from build123d import *

# Parameters (mm, degrees)
F0_R     = 12.7
F1_DEPTH = 1.27
F3_DEPTH = 25.4
F5_W     = 1.905
F5_H     = 31.75
F6_DEPTH = 6.35
F7_R     = 5.08


with BuildPart() as f1:
    # F0 (on Top) → F1 (new body)
    with BuildSketch(Plane.XY):
        Circle(F0_R)
    extrude(amount=F1_DEPTH)

    # F2 (on Top) → F3 (join)
    with BuildSketch(Plane.XY):
        Polygon((19.35988, 12.7), (-19.05, 12.7), (-19.05, -50.8), (-8.7376, -50.8), (-8.7376, -19.05), (9.0424, -19.05), (9.0424, -50.8), (19.35988, -50.8), align=None)
    extrude(amount=-F3_DEPTH)

    # F5 (on face) → F6 (cut)
    with BuildSketch(Plane(origin=(0, 0, -25.4), x_dir=(1, 0, 0), z_dir=(0, 0, -1))):
        with Locations((-9.6901, 34.925)):
            Rectangle(F5_W, F5_H)
        with Locations((9.9949, 34.925)):
            Rectangle(F5_W, F5_H)
    extrude(amount=-F6_DEPTH, mode=Mode.SUBTRACT)

    # F7
    f7_edges = [f1.edges().sort_by_distance(p)[0] for p in [
        (-13.8938, -50.8, 0),
        (-19.05, -50.8, -12.7),
        (14.20114, -50.8, 0),
        (19.35988, -50.8, -12.7),
        (19.35988, 12.7, -12.7),
        (-19.05, 12.7, -12.7),
    ]]
    fillet(f7_edges, radius=F7_R)


solid = f1.part
Part model, mm, in its own coordinate system. A direction names the side the tool comes from. Give positions to 0.01 mm unless a question says otherwise; leave off trailing zeros. Write each loop counter-clockwise with the first axis right and the second up, starting at its lowest first coordinate (ties: lowest second). Pieces come first, ordered by that corner, then holes.
1) Two-plate mould, pull along X, no slides. Class faces 1 (the face through (-2.75, -12.4, 0.63)), 2 (the face through (12, -50.8, -15)), 3 (the face through (17.832, 11.251, -12.878)), 4 (the face through (10, -35, -19.05)): released by +X, released by -X, zero draft, split by the parting line, or undercut.
Resolved:
face 1: split by the parting line
face 2: zero draft
face 3: released by +X
face 4: undercut
2) Which spindle directions (+Z, -Z, +X, -X, +Y, -Y) get a long thin tool onto all of the face, cutting with end or side? Do faces 5 (the face through (-10, -35, -19.05)), 6 (the face through (-8.738, -35, -9)), 7 (the face through (0, 0, 1.27)). Say none if no direction does.
Resolved:
face 5: -Z, -Y
face 6: +Z, -Z, -Y
face 7: +Z, +X, -X, +Y, -Y
3) Cut at A-A on y = 0. Write the cut outline in (x, z).
Resolved:
outline: (-19.05, -25.4) - (19.36, -25.4) - (19.36, 0) - (12.7, 0) - (12.7, 1.27) - (-12.7, 1.27) - (-12.7, 0) - (-19.05, 0) - close
4) Pin check, flat tips, straight feed: pin 1 (11.5 mm diameter, centred on x = -1.5, y = -22.5, fed in from +Z); pin 2 (0.6 mm diameter, centred on x = 10, y = -37, fed in from -Z); pin 3 (6.5 mm diameter, centred on x = 3, z = -7, fed in from -Y). Stop position of each tip, or through.
Resolved:
pin 1: stops at z = 0
pin 2: stops at z = -19.05
pin 3: stops at y = -19.05
5) Cut at B-B on z = -22.5. Write the cut outline in (x, y).
Resolved:
outline: (-19.05, -45.72) arc R5.08 ccw to (-13.97, -50.8) - (-10.64, -50.8) - (-10.64, -19.05) - (10.95, -19.05) - (10.95, -50.8) - (14.28, -50.8) arc R5.08 ccw to (19.36, -45.72) - (19.36, 7.62) arc R5.08 ccw to (14.28, 12.7) - (-13.97, 12.7) arc R5.08 ccw to (-19.05, 7.62) - close
6) Cut at D-D on x = -3. Write the cut outline in (y, z), then the cut area to 3 significant figures.
Resolved:
outline: (-19.05, -25.4) - (12.7, -25.4) - (12.7, 0) - (12.34, 0) - (12.34, 1.27) - (-12.34, 1.27) - (-12.34, 0) - (-19.05, 0) - close
area: 838 mm2
7) Cut at C-C on y = -43. Write the cut outline in (x, z).
Resolved:
outline: (-19.05, -25.4) - (-10.64, -25.4) - (-10.64, -19.05) - (-8.74, -19.05) - (-8.74, 0) - (-19.05, 0) - close; (9.04, -19.05) - (10.95, -19.05) - (10.95, -25.4) - (19.36, -25.4) - (19.36, 0) - (9.04, 0) - close
8) Probe L1, parallel to X at y = -31.5, z = -17.25; L2, parallel to X at y = -34, z = -23.75; L3, parallel to Y at x = -6.5, z = -1.5. List the from-to ranges inside material, lowest first.
Resolved:
L1: x = -19.05 to -8.74, 9.04 to 19.36
L2: x = -19.05 to -10.64, 10.95 to 19.36
L3: y = -19.05 to 12.7
